Can you work these out from the model? Positions are in its coordinate system, mm. Face numbers are marked on the shaded views. A direction names the side the tool comes from. Give positions to 0.01 mm unless a question says otherwise; leave off trailing zeros. Write each loop counter-clockwise with the first axis right and the second up, starting at its lowest first coordinate (ties: lowest second). Pieces come first, ordered by that corner, then holes.
```python
from build123d import *

# Parameters (mm, degrees)
SM_BASE_FLANGE_1_DEPTH      = 30
SM_EDGE_FLANGE_1_DEPTH      = 25
SM_EDGE_FLANGE_1_BEND_DEPTH = 25
SKETCH_10_R                 = 4.05
CUT_EXTRUDE_1_DEPTH         = 79.198465458
SKETCH_11_R                 = 4.05
CUT_EXTRUDE_2_DEPTH         = 84.054199171
FILLET_1_R                  = 6
SKETCH_12_W                 = 8.2
SKETCH_12_H                 = 8.2
CUT_EXTRUDE_3_DEPTH         = 4
SM_BASE_FLANGE_1_2_DEPTH    = 4
SM_BASE_FLANGE_2_DEPTH      = 4
FILLET_2_R                  = 15
FILLET_3_R                  = 2


# Sheet-metal steps are written as plain solids
with BuildPart() as part:
    # Sketch 1 → Sm Base Flange 1 (new body)
    with BuildSketch(Plane(origin=(0, 0, 0), x_dir=(0, 0, -1), z_dir=(1, 0, 0))):
        with BuildLine():
            Line((25, -63), (9, -63))
            ThreePointArc((9, -63), (2.636038969, -60.363961031), (0, -54))
            Line((0, -54), (0, -9))
            ThreePointArc((0, -9), (2.636038969, -2.636038969), (9, 0))
            Line((9, 0), (25, 0))
            Line((25, 0), (25, -4))
            Line((25, -4), (9, -4))
            ThreePointArc((9, -4), (5.464466094, -5.464466094), (4, -9))
            Line((4, -9), (4, -54))
            ThreePointArc((4, -54), (5.464466094, -57.535533906), (9, -59))
            Line((9, -59), (25, -59))
            Line((25, -59), (25, -63))
        make_face()
    extrude(amount=SM_BASE_FLANGE_1_DEPTH)

    # Ребро-кромка1 section (across the edge) → Ребро-кромка1 (add)
    with BuildSketch(Plane(origin=(-5, -19, 0), x_dir=(1, 0, 0), z_dir=(0, -1, 0))):
        with BuildLine():
            Line((-4, 5), (-4, 25))
            Line((-4, 25), (0, 25))
            Line((0, 25), (0, 5))
            ThreePointArc((0, 5), (1.464466094, 1.464466094), (5, 0))
            Line((5, 0), (5, -4))
            ThreePointArc((5, -4), (-1.363961031, -1.363961031), (-4, 5))
        make_face()
    extrude(amount=SM_EDGE_FLANGE_1_DEPTH)

    # Ребро-кромка1 section 2 (across the edge) → Ребро-кромка1 bend (add)
    with BuildSketch(Plane(origin=(35, -44, 0), x_dir=(-1, 0, 0), z_dir=(0, 1, 0))):
        with BuildLine():
            Line((-4, 5), (-4, 25))
            Line((-4, 25), (0, 25))
            Line((0, 25), (0, 5))
            ThreePointArc((0, 5), (1.464466094, 1.464466094), (5, 0))
            Line((5, 0), (5, -4))
            ThreePointArc((5, -4), (-1.363961031, -1.363961031), (-4, 5))
        make_face()
    extrude(amount=SM_EDGE_FLANGE_1_BEND_DEPTH)

    # Эскиз10 → Вырез-Вытянуть1 (cut, through all)
    with BuildSketch(Plane(origin=(0, 0, 0), x_dir=(1, 0, 0), z_dir=(0, 1, 0))):
        with Locations(Location((15, 17, 0), (0, 0, 270))):
            Circle(SKETCH_10_R)
    extrude(amount=-CUT_EXTRUDE_1_DEPTH, mode=Mode.SUBTRACT)

    # Эскиз11 → Вырез-Вытянуть2 (cut, through all)
    with BuildSketch(Plane(origin=(39, 0, 0), x_dir=(0, 0, -1), z_dir=(1, 0, 0))):
        with Locations((-15, -31.5)):
            Circle(SKETCH_11_R)
    extrude(amount=-CUT_EXTRUDE_2_DEPTH, mode=Mode.SUBTRACT)

    # Скругление1
    fillet_1_edges = [part.edges().sort_by_distance(p)[0] for p in [
        (0, -61, -25),
        (0, -2, -25),
        (30, -61, -25),
        (30, -2, -25),
    ]]
    fillet(fillet_1_edges, radius=FILLET_1_R)

    # Эскиз12 → Вырез-Вытянуть3 (cut)
    with BuildSketch(Plane(origin=(0, 0, 0), x_dir=(1, 0, 0), z_dir=(0, 1, 0))):
        with Locations((15, 17)):
            Rectangle(SKETCH_12_W, SKETCH_12_H)
    extrude(amount=-CUT_EXTRUDE_3_DEPTH, mode=Mode.SUBTRACT)

    # Эскиз13 → Sm Base Flange 1 2 (add)
    with BuildSketch(Plane(origin=(39, 0, 0), x_dir=(0, 0, -1), z_dir=(1, 0, 0))):
        Polygon((-25, -19), (-23.891346313, 1), (-30.590076124, -24), (-30.590076124, -39), (-23.891346313, -64), (-25, -44), align=None)
    extrude(amount=-SM_BASE_FLANGE_1_2_DEPTH)

    # Эскиз14 → Выступ2 (add)
    with BuildSketch(Plane.ZY.offset(9)):
        Polygon((25, -19), (23.891346313, 1), (30.590076124, -24), (30.590076124, -39), (23.891346313, -64), (25, -44), align=None)
    extrude(amount=-SM_BASE_FLANGE_2_DEPTH)

    # Скругление2
    fillet_2_edges = [part.edges().sort_by_distance(p)[0] for p in [
        (37, -39, 30.590076124),
        (37, -24, 30.590076124),
        (-7, -24, 30.590076124),
        (-7, -39, 30.590076124),
        (-7, -19, 25),
        (-7, -44, 25),
        (37, -44, 25),
        (37, -19, 25),
    ]]
    fillet(fillet_2_edges, radius=FILLET_2_R)

    # Скругление3
    fillet_3_edges = [part.edges().sort_by_distance(p)[0] for p in [
        (-7, -64, 23.891346313),
        (37, -64, 23.891346313),
        (37, 1, 23.891346313),
        (-7, 1, 23.891346313),
    ]]
    fillet(fillet_3_edges, radius=FILLET_3_R)


solid = part.part
```
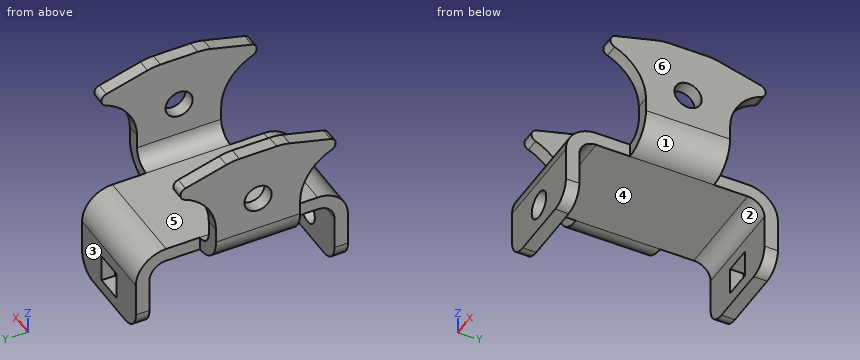
1) Suppose I cut it at A-A on x = 15. Write out the boundary of the cut face in (y, z), plus the area to 3 significant figures.
Values follow:
outline: (-63, -25) - (-59, -25) - (-59, -21.05) - (-63, -21.05) - close; (-63, -12.95) - (-59, -12.95) - (-59, -9) arc R5 cw to (-54, -4) - (-9, -4) arc R5 cw to (-4, -9) - (-4, -12.9) - (0, -12.9) - (0, -9) arc R9 ccw to (-9, 0) - (-54, 0) arc R9 ccw to (-63, -9) - close; (-4, -25) - (0, -25) - (0, -21.1) - (-4, -21.1) - close
area: 331 mm2
2) Suppose I cut it at D-D on z = -10.5. Write out the boundary of the cut face in (x, y).
Values follow:
outline: (0, -63) - (30, -63) - (30, -59) - (0, -59) - close; (0, -4) - (30, -4) - (30, 0) - (0, 0) - close
3) Suppose I cut it at B-B on z = -17. Write out the boundary of the cut face in (x, y), plus the area to 3 significant figures.
Values follow:
outline: (0, -63) - (10.95, -63) - (10.95, -59) - (0, -59) - close; (0, -4) - (10.9, -4) - (10.9, 0) - (0, 0) - close; (19.05, -63) - (30, -63) - (30, -59) - (19.05, -59) - close; (19.1, -4) - (30, -4) - (30, 0) - (19.1, 0) - close
area: 175 mm2
4) Please list where these lines run through material, in increasing order: L1, parallel to X at y = -29, z = 22.5; L2, parallel to X at y = -61, z = -17; L3, parallel to Y at x = 28.5, z = -18.
Values follow:
L1: x = -9 to -5, 35 to 39
L2: x = 0 to 10.95, 19.05 to 30
L3: y = -63 to -59, -4 to 0
5) For the marked faces 4, 5 and 6, which set-ups out of +Z, -Z, +X, -X, +Y, -Y let a thin tool reach every point of the face, with its end or its side?
Values follow:
face 4: -Z, +X, -X
face 5: +Z, +Y, -Y
face 6: +Z, -Z, +X, +Y, -Y
6) Suppose I cut it at C-C on y = -31.5. Write out the boundary of the cut face in (x, z).
Values follow:
outline: (-9, 5) arc R9 ccw to (0, -4) - (30, -4) arc R9 ccw to (39, 5) - (39, 10.95) - (35, 10.95) - (35, 5) arc R5 cw to (30, 0) - (0, 0) arc R5 cw to (-5, 5) - (-5, 10.95) - (-9, 10.95) - close; (-9, 19.05) - (-5, 19.05) - (-5, 30.59) - (-9, 30.59) - close; (35, 19.05) - (39, 19.05) - (39, 30.59) - (35, 30.59) - close
7) If we mould it in two halves opening along Y, with no side actions, what happens to the marked faces 1, 2 and 3? For each: +Y half, -Y half, draft (parallel to the pull), parting line (faces both ways), or undercut.
Values follow:
face 1: draft
face 2: undercut
face 3: +Y half
8) For pin 1 Ø3 at (y, z) = (-37.5, 0.5) entering from -X; pin 2 Ø5 at (x, y) = (8.5, -54) entering from +Z; pin 3 Ø15 at (y, z) = (-53.5, -6.5) entering from +X, each with a flat end and sliding along its axis, tell me the tip position at first contact or that it passes through.
Values follow:
pin 1: stops at x = -8.49
pin 2: stops at z = 0
pin 3: stops at x = 30
